Autodesk Fusion 360 part; units mm, degrees
sketch "Sketch1" plane through (0, 0, 0) normal (0, 0, 1) x (1, 0, 0)
  line L0 (0, 0) -> (0, 100.5)
  line L1 (0, 100.5) -> (4.8, 100.5)
  line L2 (4.8, 100.5) -> (4.8, 98.25)
  line L3 (4.8, 98.25) -> (4.5, 98.25)
  line L4 (4.5, 98.25) -> (4.5, 81.7479)
  line L5 (10.2824, 61.4) -> (10.2824, 5.2127)
  line L6 (0, 0) -> (8.8361, 0)
  arc A0 (8.8361, 0) -> (10.2824, 5.2127) centre (0.1654, 5.2127) ccw
  arc A1 (4.5, 81.7479) -> (6.5345, 72.2453) centre (27.709, 81.7479) ccw
  line L7 (10.2054, 65.5631) -> (10.2824, 61.4)
  arc A2 (6.5345, 72.2453) -> (7.5928, 71.4184) centre (7.5928, 72.509) ccw
  arc A3 (10.2054, 65.5631) -> (7.5928, 71.4184) centre (1.998, 65.4114) ccw
  line L8 (8.5816, 71.4184) -> (8.683, 71.4184)
  dimension "d1" = 100.5
  dimension "d2" = 4.8
  dimension "d3" = 2.25
  dimension "d4" = 0.3
  dimension "d5" = 16.5021
  dimension "d13" = 61.4
revolve "Revolve1" add sketch "Sketch1" angle 360 about axis through (0, 0, 0) along (0, 1, 0)
equation "d1 = haed_flosku"
equation "d5 = d1 * 0.1642"
equation "d13 = d1 - 39.1 mm"
equation "haed_flosku = 100.5 mm"
Work out the finished part from the listing and answer in its coordinate system (mm). A direction names the side the tool comes from. Give positions to 0.01 mm unless a question says otherwise; leave off trailing zeros. Write each loop counter-clockwise with the first axis right and the second up, starting at its lowest first coordinate (ties: lowest second). Pieces come first, ordered by that corner, then holes. Notation, with made-up numbers: (2.25, 44) - (16.25, 44) arc R35 cw to (16.25, 82) - close; hole circle Ø8 at (27, 4). An arc over 180 degrees is marked (long way). One line per item, written item: value. Start each with the question number.
1. Find section A-A (y = 53). Write down the section's boundary in (x, z), then the cut area to 3 significant figures.
2. For faces 4 (the cylindrical face through (-2.229, 32.913, -10.038)), 5 (the conical face through (-2.22, 63.45, -10)), determine the directions among +Z, -Z, +X, -X, +Y, -Y from which every point of the face is accessible in a straight line to the end or side of a thin tool.
3. Consider probe 1 along X at (y, z) = (6, -8); probe 2 along X at (y, z) = (35.5, -2.25); probe 3 along Y at (x, z) = (-7.75, 3.5). Determine where each line is inside the solid, lowest interval first.
4. For a pull along Y with two mould halves and no side action, classify faces 1 (the cylindrical face through (-0.59, 89.88, 4.46)), 2 (the flat face through (0, 100.5, 0)), 3 (the flat face through (0, 0, 0)) as +Y half, -Y half, draft (parallel to the pull), parting line (faces both ways), or undercut.
5. Given pin 1 (3 mm diameter, centred on x = -0.5, z = 0, fed in from -Y); pin 2 (2 mm diameter, centred on x = -8, z = 0.5, fed in from +Y); pin 3 (2 mm diameter, centred on y = 30, z = -2, fed in from +X); pin 4 (1 mm diameter, centred on y = 66.5, z = 3.5, fed in from +X), each flat-ended and moving along its own axis, determine where each tip first touches the part or whether it passes through.
6. Find section B-B (y = 83.5). Write down the section's boundary in (x, z), then the cut area to 3 significant figures.
Geometry results:
1. outline: circle Ø20.56 at (0, 0)
1. area: 332 mm2
2. face 4: +Y, -Y
2. face 5: +Y
3. probe 1: -6.46 to 6.46
3. probe 2: -10.03 to 10.03
3. probe 3: 0 to 70.42
4. face 1: undercut
4. face 2: +Y half
4. face 3: -Y half
5. pin 1: y = 0
5. pin 2: y = 71.58
5. pin 3: x = 10.23
5. pin 4: x = 9.69
6. outline: circle Ø9 at (0, 0)
6. area: 63.6 mm2
